Read the model definition and answer for the solid it produces. Units are mm, in the model's axes. Face numbers are marked on the shaded views. Coordinates: 2 decimals unless noted, no trailing zeros. Write each loop counter-clockwise with the first axis right and the second up, starting at its lowest first coordinate (ties: lowest second). Pieces come first, ordered by that corner, then holes. Notation, with made-up numbers: (74, -25.75) -> (123, -25.75) arc R29 ccw to (123, 8.25) -> close; hole circle Ø9 at (-3, 74). An arc over 180 degrees is marked (long way). Answer in a Markdown table with one row per item. Add a question column.
Item 1: Given pin 1 Ø2 at (y, z) = (-5.5, 5.5) entering from -X; pin 2 Ø1.5 at (y, z) = (-7, 14.5) entering from -X; pin 3 Ø6 at (y, z) = (3.5, 5.5) entering from +X, each flat-ended and moving along its own axis, determine where each tip first touches the part or whether it passes through.
Item 2: Section B-B on z = 19.75 is taken. Write down the section's boundary in (x, y), then the cut area to 3 significant figures.
Item 3: Straight lines are drawn through the part: line 1 (Y direction, x = 0, z = 7); line 2 (Z direction, x = 0.5, y = 4.5); line 3 (Y direction, x = 0, z = 19.6). For each, find the intervals that lie inside material, in ascending order. Write a range as from..to.
Item 4: Section C-C on z = 11.5 is taken. Write down the section's boundary in (x, y).
Item 5: Section A-A on x = 0 is taken. Write down the section's boundary in (y, z), then the cut area to 3 significant figures.
Item 6: For a pull along Y with two mould halves and no side action, classify the marked faces 1, 2 and 3 as +Y half, -Y half, draft (parallel to the pull), parting line (faces both ways), or undercut.
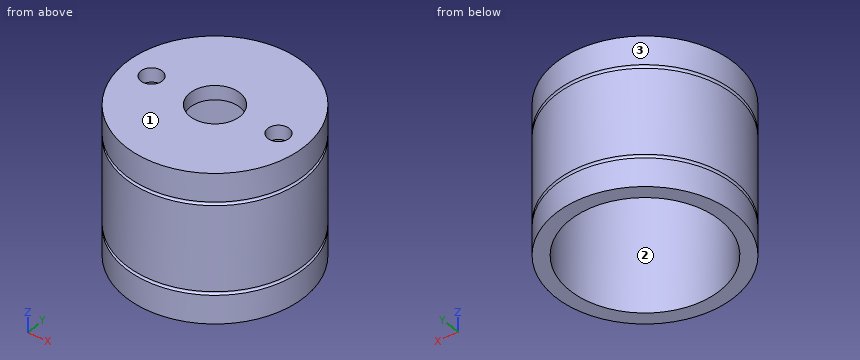
```python
from build123d import *

# Parameters (mm, degrees)
SKETCH1_R           = 12.5
BOSS_EXTRUDE1_DEPTH = 21
SHELL1_T            = -2
SKETCH3_R           = 3.5
CUT_EXTRUDE1_DEPTH  = 28.449954463
SKETCH4_R           = 1.5
CUT_EXTRUDE2_DEPTH  = 28.449954463
SKETCH9_R           = 0.25
SKETCH8_R           = 0.25


with BuildPart() as part:
    # Sketch1 → Boss-Extrude1 (new body)
    with BuildSketch(Plane.XY):
        with Locations(Location((0, 0, 0), (0, 0, 180))):
            Circle(SKETCH1_R)
    extrude(amount=BOSS_EXTRUDE1_DEPTH)

    # Shell1
    shell1_openings = [part.faces().sort_by_distance(p)[0] for p in [
        (0, 0, 0),
    ]]
    offset(amount=SHELL1_T, openings=shell1_openings, kind=Kind.INTERSECTION)

    # Sketch3 → Cut-Extrude1 (cut, through all)
    with BuildSketch(Plane.XY.offset(21)):
        Circle(SKETCH3_R)
    extrude(amount=-CUT_EXTRUDE1_DEPTH, mode=Mode.SUBTRACT)

    # Sketch4 → Cut-Extrude2 (cut, through all)
    with BuildSketch(Plane.XY.offset(21)):
        with Locations((8.75, 0)):
            Circle(SKETCH4_R)
        with Locations((-8.75, 0)):
            Circle(SKETCH4_R)
    extrude(amount=-CUT_EXTRUDE2_DEPTH, mode=Mode.SUBTRACT)

    # Cut-Sweep1: sweep along a path in Sketch6
    with BuildLine(Plane.XY.offset(16.75)) as cut_sweep1_path:
        CenterArc((0, 0), 12.5, 0, 360)
    # Sketch9 → Cut-Sweep1 (sweep, cut)
    with BuildSketch(Plane(origin=(0, 0, 0), x_dir=(0, 0, -1), z_dir=(1, 0, 0))):
        with Locations((-16.75, 12.5)):
            Circle(SKETCH9_R)
    sweep(path=cut_sweep1_path.line, mode=Mode.SUBTRACT)

    # Cut-Sweep2: sweep along a path in Sketch7
    with BuildLine(Plane(origin=(0, 0, 4.25), x_dir=(-1, 0, 0), z_dir=(0, 0, -1))) as cut_sweep2_path:
        CenterArc((0, 0), 12.5, 0, 360)
    # Sketch8 → Cut-Sweep2 (sweep, cut)
    with BuildSketch(Plane(origin=(0, 0, 0), x_dir=(0, 0, -1), z_dir=(1, 0, 0))):
        with Locations((-4.25, 12.5)):
            Circle(SKETCH8_R)
    sweep(path=cut_sweep2_path.line, mode=Mode.SUBTRACT)


solid = part.part
```
Results below:
| question | item | result |
|---|---|---|
| 1 | pin 1 | stops at x = -11.66 |
| 1 | pin 2 | stops at x = -10.83 |
| 1 | pin 3 | stops at x = 12.49 |
| 2 | outline | circle Ø25 at (0, 0); hole circle Ø3 at (-8.75, 0); hole circle Ø7 at (0, 0); hole circle Ø3 at (8.75, 0) |
| 2 | area | 438 mm2 |
| 3 | line 1 | y = -12.5..-10.5, 10.5..12.5 |
| 3 | line 2 | z = 19..21 |
| 3 | line 3 | y = -12.5..-3.5, 3.5..12.5 |
| 4 | outline | circle Ø25 at (0, 0); hole circle Ø21 at (0, 0) |
| 5 | outline | (-12.5, 0) -> (-10.5, 0) -> (-10.5, 19) -> (-3.5, 19) -> (-3.5, 21) -> (-12.5, 21) -> (-12.5, 17) arc R0.25 cw to (-12.5, 16.5) -> (-12.5, 4.5) arc R0.25 cw to (-12.5, 4) -> close; (3.5, 19) -> (10.5, 19) -> (10.5, 0) -> (12.5, 0) -> (12.5, 4) arc R0.25 cw to (12.5, 4.5) -> (12.5, 16.5) arc R0.25 cw to (12.5, 17) -> (12.5, 21) -> (3.5, 21) -> close |
| 5 | area | 112 mm2 |
| 6 | face 1 | draft |
| 6 | face 2 | undercut |
| 6 | face 3 | parting line |
